from build123d import *

# Parameters (mm, degrees)
ESBO_O1_W                        = 120
ESBO_O1_H                        = 15
FLANGE_BASE1_DEPTH               = 1.2
ARESTA_FLANGE1_STRIP_W           = 8.8
ARESTA_FLANGE1_STRIP_H           = 1.2
ARESTA_FLANGE1_STRIP_CUT_DEPTH   = 15
ARESTA_FLANGE1_STRIP_2_W         = 8.8
ARESTA_FLANGE1_STRIP_2_H         = 1.2
ARESTA_FLANGE1_STRIP_CUT_2_DEPTH = 15
ARESTA_FLANGE1_DEPTH             = 15
ARESTA_FLANGE1_BEND_DEPTH        = 15
QUEBRA_CANTO1_DEPTH              = 120
FURO_DE_DI_METRO_3_5_3_5_1_D     = 3.5
FURO_DE_DI_METRO_3_5_3_5_1_DEPTH = 1.2
FURO_DE_DI_METRO_3_5_3_5_2_D     = 3.5


# Read off the part's stored shape, not the designer's step: Quebra-Canto1
# Sheet-metal steps are written as plain solids
with BuildPart() as part:
    # Esboço1 → Flange-base1 (new body)
    with BuildSketch(Plane.XY):
        with Locations((60, 7.5)):
            Rectangle(ESBO_O1_W, ESBO_O1_H)
    extrude(amount=-FLANGE_BASE1_DEPTH)

    # Aresta-Flange1 strip (across the edge) → Aresta-Flange1 strip cut (cut)
    with BuildSketch(Plane(origin=(120, 15, -1.2), x_dir=(-1, 0, 0), z_dir=(0, -1, 0))):
        with Locations((-1.2, -0.6)):
            Rectangle(ARESTA_FLANGE1_STRIP_W, ARESTA_FLANGE1_STRIP_H)
    extrude(amount=ARESTA_FLANGE1_STRIP_CUT_DEPTH, mode=Mode.SUBTRACT)

    # Aresta-Flange1 strip 2 (across the edge) → Aresta-Flange1 strip cut 2 (cut)
    with BuildSketch(Plane(origin=(0, 0, -1.2), x_dir=(1, 0, 0), z_dir=(0, 1, 0))):
        with Locations((-1.2, -0.6)):
            Rectangle(ARESTA_FLANGE1_STRIP_2_W, ARESTA_FLANGE1_STRIP_2_H)
    extrude(amount=ARESTA_FLANGE1_STRIP_CUT_2_DEPTH, mode=Mode.SUBTRACT)

    # Aresta-Flange1 section (across the edge) → Aresta-Flange1 (add)
    with BuildSketch(Plane(origin=(120, 15, -1.2), x_dir=(-1, 0, 0), z_dir=(0, -1, 0))):
        with BuildLine():
            Line((0, 2), (0, 13.8))
            Line((0, 13.8), (1.2, 13.8))
            Line((1.2, 13.8), (1.2, 2))
            ThreePointArc((1.2, 2), (1.785786438, 0.585786438), (3.2, 0))
            Line((3.2, 0), (3.2, -1.2))
            ThreePointArc((3.2, -1.2), (0.9372583, -0.2627417), (0, 2))
        make_face()
    extrude(amount=ARESTA_FLANGE1_DEPTH)

    # Aresta-Flange1 section 2 (across the edge) → Aresta-Flange1 bend (add)
    with BuildSketch(Plane(origin=(0, 0, -1.2), x_dir=(1, 0, 0), z_dir=(0, 1, 0))):
        with BuildLine():
            Line((0, 2), (0, 13.8))
            Line((0, 13.8), (1.2, 13.8))
            Line((1.2, 13.8), (1.2, 2))
            ThreePointArc((1.2, 2), (1.785786438, 0.585786438), (3.2, 0))
            Line((3.2, 0), (3.2, -1.2))
            ThreePointArc((3.2, -1.2), (0.9372583, -0.2627417), (0, 2))
        make_face()
    extrude(amount=ARESTA_FLANGE1_BEND_DEPTH)

    # Quebra-Canto1 outline → Quebra-Canto1 (cut)
    with BuildSketch(Plane.YZ):
        with BuildLine():
            Line((15, -15), (15, -10))
            ThreePointArc((15, -10), (13.535533906, -13.535533906), (10, -15))
            Line((10, -15), (15, -15))
        make_face()
        with BuildLine():
            Line((0, -15), (5, -15))
            ThreePointArc((5, -15), (1.464466094, -13.535533906), (0, -10))
            Line((0, -10), (0, -15))
        make_face()
    extrude(amount=QUEBRA_CANTO1_DEPTH, mode=Mode.SUBTRACT)

    # Furo de diâmetro Ø3.5 (3.5)1
    with Locations(Plane(origin=(120, 0, 0), x_dir=(0, 0, -1), z_dir=(1, 0, 0))):
        with Locations((8, 7.5)):
            Hole(FURO_DE_DI_METRO_3_5_3_5_1_D / 2, depth=FURO_DE_DI_METRO_3_5_3_5_1_DEPTH)

    # Furo de diâmetro Ø3.5 (3.5)2 (through all)
    with Locations(Plane.ZY):
        with Locations((-8, 7.5)):
            Hole(FURO_DE_DI_METRO_3_5_3_5_2_D / 2)


solid = part.part
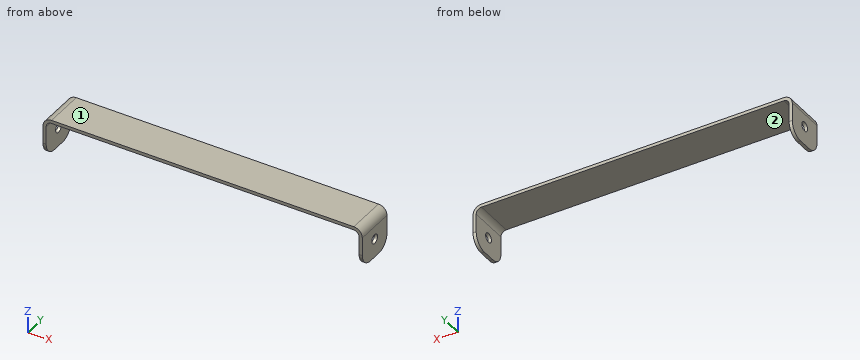
Can you work these out from the model? Positions are in its coordinate system, mm. Face numbers are marked on the shaded views. Round coordinates to 2 decimals unless told otherwise and drop trailing zeros. Write each loop counter-clockwise with the first axis right and the second up, starting at its lowest first coordinate (ties: lowest second). Pieces come first, ordered by that corner, then holes. Notation, with made-up numbers: M 79,18 L 86,18 A20 ccw 86,34 Z; hole C 36.25,-2.5 d5. An arc over 180 degrees is marked long. Use a Markdown table: item, result.
Item 1: I want a section at C-C (z = -13). List the corners of the cut face in (x, y) for me.
Found:
| item | result |
|---|---|
| outline | M 0,1 L 1.2,1 L 1.2,14 L 0,14 Z; M 118.8,1 L 120,1 L 120,14 L 118.8,14 Z |
Item 2: We'd pull the mould along X, two halves only. Please class the marked faces 1 and 2: released by +X, released by -X, zero draft, split by the parting line, or undercut.
Found:
| item | result |
|---|---|
| face 1 | zero draft |
| face 2 | undercut |
Item 3: For pin 1 Ø8 at (y, z) = (6.5, -7) entering from -X; pin 2 Ø7.5 at (x, y) = (53.5, 7.5) entering from -Z; pin 3 Ø2 at (y, z) = (7.5, -8) entering from -X (3 decimals), each with a flat end and sliding along its axis, tell me the tip position at first contact or that it passes through.
Found:
| item | result |
|---|---|
| pin 1 | stops at x = 0 |
| pin 2 | stops at z = -1.2 |
| pin 3 | passes through |
Item 4: I want a section at B-B (z = -8). List the corners of the cut face in (x, y) for me.
Found:
| item | result |
|---|---|
| outline | M 0,0 L 1.2,0 L 1.2,5.75 L 0,5.75 Z; M 0,9.25 L 1.2,9.25 L 1.2,15 L 0,15 Z; M 118.8,0 L 120,0 L 120,5.75 L 118.8,5.75 Z; M 118.8,9.25 L 120,9.25 L 120,15 L 118.8,15 Z |
Item 5: If I drill on line 1 along X through (y, z) = (12.5, -10.75); line 2 along Y through (x, z) = (119.4, -8); line 3 along Z through (x, y) = (9, 7.5), over which ranges is the centre line in solid material (lowest first)? Write a range as [from, to].
Found:
| item | result |
|---|---|
| line 1 | x = [0, 1.2], [118.8, 120] |
| line 2 | y = [0, 5.75], [9.25, 15] |
| line 3 | z = [-1.2, 0] |
Item 6: I want a section at D-D (x = 24.5). List the corners of the cut face in (y, z) for me, and give its area (3 significant figures).
Found:
| item | result |
|---|---|
| outline | M 0,-1.2 L 15,-1.2 L 15,0 L 0,0 Z |
| area | 18.0 mm2 |
Item 7: I want a section at A-A (y = 7.5). List the corners of the cut face in (x, z) for me, and give its area (3 significant figures).
Found:
| item | result |
|---|---|
| outline | M 0,-15 L 1.2,-15 L 1.2,-9.75 L 0,-9.75 Z; M 0,-6.25 L 1.2,-6.25 L 1.2,-3.2 A2 cw 3.2,-1.2 L 116.8,-1.2 A2 cw 118.8,-3.2 L 118.8,-6.25 L 120,-6.25 L 120,-3.2 A3.2 ccw 116.8,0 L 3.2,0 A3.2 ccw 0,-3.2 Z; M 118.8,-15 L 120,-15 L 120,-9.75 L 118.8,-9.75 Z |
| area | 166 mm2 |
